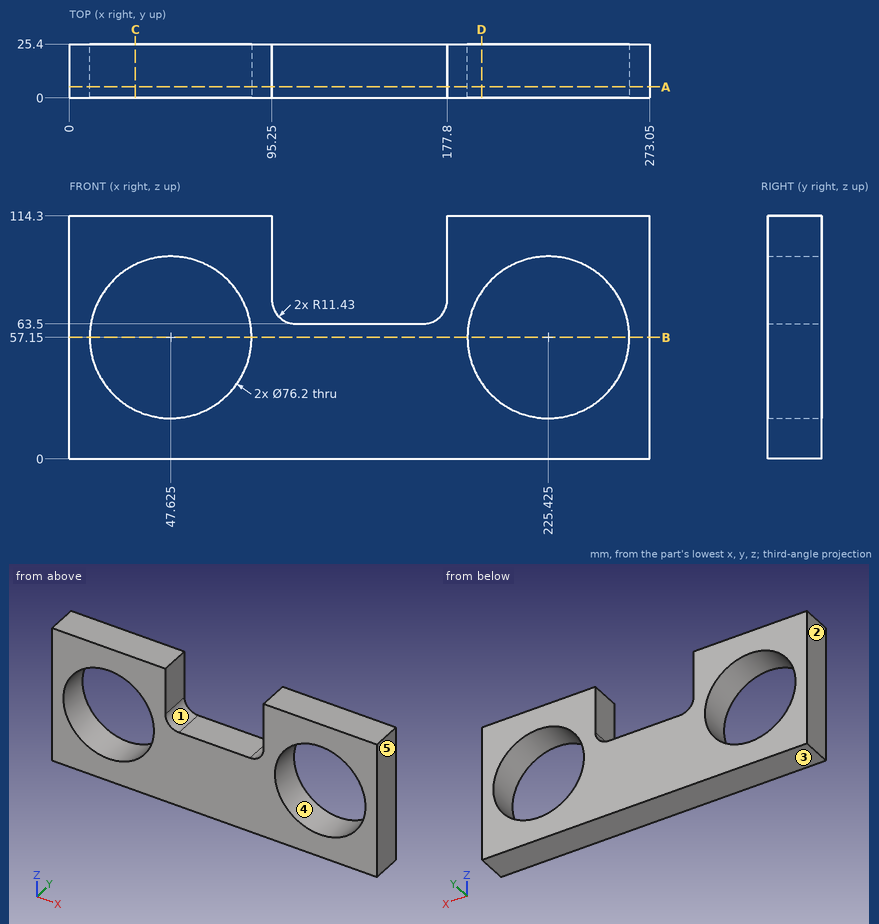
Source: three-view drawing plus pictorial views. Frame: mm from the lowest corner of the part. A direction names the side the tool comes from. Coordinates: 2 decimals unless noted, no trailing zeros. Order: outer loops, then holes, each group sorted by start corner. A loop starts at its lowest first (then second) coordinate and runs counter-clockwise, first axis right, second up.
Item 1: Cut plane B-B (z = 57.15). Return loops of the section in (x, y) (3 decimals), plus the area to 3 significant figures.
Output values:
outline: (0, 0) - (9.525, 0) - (9.525, 25.4) - (0, 25.4) - close; (85.725, 0) - (187.325, 0) - (187.325, 25.4) - (85.725, 25.4) - close; (263.525, 0) - (273.05, 0) - (273.05, 25.4) - (263.525, 25.4) - close
area: 3,060 mm2
Item 2: Set-up query: the marked faces 1 and 2. Return all of +Z, -Z, +X, -X, +Y, -Y with unobstructed straight access to the full face (end or side cutting, diameter ignored); none if empty.
Output values:
face 1: +Z, +Y, -Y
face 2: +Z, -Z, -X, +Y, -Y
Item 3: Cut plane C-C (x = 31). Return loops of the section in (y, z).
Output values:
outline: (0, 0) - (25.4, 0) - (25.4, 22.87) - (0, 22.87) - close; (0, 91.43) - (25.4, 91.43) - (25.4, 114.3) - (0, 114.3) - close
Item 4: First-contact query: P1, Ø12, axis at y = 11.5, z = 92.5, coming from the -X side; P2, Ø1.5, axis at x = 154, y = 22, coming from the +Z side; P3, Ø10, axis at x = 73.5, z = 75.5, coming from the -Y side. Flat tips, straight axial feed; report the tip coordinate or a pass-through.
Output values:
P1: stops at x = 0
P2: stops at z = 63.5
P3: passes through
Item 5: Cut plane A-A (y = 5.25). Return loops of the section in (x, z) (3 decimals), plus the area to 3 significant figures.
Output values:
outline: (0, 0) - (273.05, 0) - (273.05, 114.3) - (177.8, 114.3) - (177.8, 74.93) arc R11.43 cw to (166.37, 63.5) - (106.68, 63.5) arc R11.43 cw to (95.25, 74.93) - (95.25, 114.3) - (0, 114.3) - close; hole circle Ø76.2 at (47.625, 57.15); hole circle Ø76.2 at (225.425, 57.15)
area: 18,000 mm2
Item 6: Pull-direction query (X, two-part tool) for the marked faces 3, 4 and 5; classes: pulls with the +X half, pulls with the -X half, needs draft (parallel to the pull), parting line crosses it, or undercut.
Output values:
face 3: needs draft
face 4: undercut
face 5: pulls with the +X half
Item 7: Cut plane D-D (x = 194). Return loops of the section in (y, z).
Output values:
outline: (0, 0) - (25.4, 0) - (25.4, 35.61) - (0, 35.61) - close; (0, 78.69) - (25.4, 78.69) - (25.4, 114.3) - (0, 114.3) - close
Item 8: Material intervals for line 1 (X direction, y = 13, z = 57.5); line 2 (Z direction, x = 49.5, y = 2); line 3 (X direction, y = 2.5, z = 68), sorted ascending.
Output values:
line 1: x = 0 to 9.53, 85.72 to 187.33, 263.52 to 273.05
line 2: z = 0 to 19.1, 95.2 to 114.3
line 3: x = 0 to 11.1, 84.15 to 97.59, 175.46 to 188.9, 261.95 to 273.05
